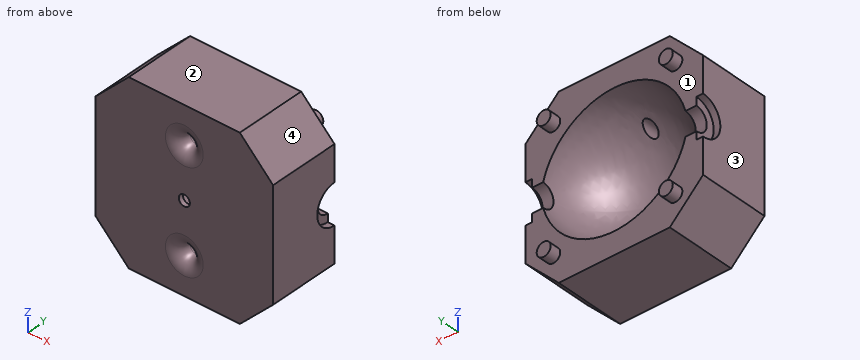
from build123d import *

# Parameters (mm, degrees)
SKETCH1_W           = 80
SKETCH1_H           = 80
BOSS_EXTRUDE1_DEPTH = 32
SKETCH3_R           = 5.375
CUT_EXTRUDE1_DEPTH  = 95.994736856
CHAMFER1_SIZE       = 15
SKETCH5_R           = 9
CUT_EXTRUDE3_DEPTH  = 93.482430925
SKETCH4_R           = 3.15
BOSS_EXTRUDE3_DEPTH = 5
CUT_EXTRUDE4_REACH  = 69.594
SKETCH6_R           = 2.5
FILLET1_R           = 6


with BuildPart() as part:
    # Sketch1 → Boss-Extrude1 (new body)
    with BuildSketch(Plane(origin=(0, 0, 0), x_dir=(1, 0, 0), z_dir=(0, 1, 0))):
        Rectangle(SKETCH1_W, SKETCH1_H)
    extrude(amount=BOSS_EXTRUDE1_DEPTH)

    # Sketch2 → Cut-Revolve1 (revolve, cut)
    with BuildSketch(Plane(origin=(0, 32, 0), x_dir=(1, 0, 0), z_dir=(0, 1, 0))):
        with BuildLine():
            Line((-33, 0), (33, 0))
            ThreePointArc((33, 0), (0, -30), (-33, 0))
        make_face()
    revolve(axis=Axis((-33, 32, 0), (1, 0, 0)), mode=Mode.SUBTRACT)

    # Sketch3 → Cut-Extrude1 (cut, through all)
    with BuildSketch(Plane.ZY.offset(40)):
        with Locations((0, 32)):
            Circle(SKETCH3_R)
    extrude(amount=-CUT_EXTRUDE1_DEPTH, mode=Mode.SUBTRACT)

    # Chamfer1
    chamfer1_edges = [part.edges().sort_by_distance(p)[0] for p in [
        (40, 16, 40),
        (-40, 16, 40),
        (-40, 16, -40),
        (40, 16, -40),
    ]]
    chamfer(chamfer1_edges, length=CHAMFER1_SIZE)

    # Sketch5 → Cut-Extrude3 (cut, through all)
    with BuildSketch(Plane.ZY.offset(37)):
        with Locations((0, 32)):
            Circle(SKETCH5_R)
    cut_extrude3 = extrude(amount=CUT_EXTRUDE3_DEPTH, mode=Mode.SUBTRACT)

    # Mirror1: Cut-Extrude3 across plane
    add(cut_extrude3.mirror(Plane(origin=(0, 0, 0), x_dir=(0, 0, 1), z_dir=(1, 0, 0))), mode=Mode.SUBTRACT)

    # Sketch4 → Boss-Extrude3 (add)
    with BuildSketch(Plane(origin=(0, 32, 0), x_dir=(1, 0, 0), z_dir=(0, 1, 0))):
        with Locations(Location((-27.5, 27.5, 0), (0, 0, 270))):
            Circle(SKETCH4_R)
        with Locations(Location((27.5, 27.5, 0), (0, 0, 270))):
            Circle(SKETCH4_R)
        with Locations(Location((27.5, -27.5, 0), (0, 0, 270))):
            Circle(SKETCH4_R)
        with Locations(Location((-27.5, -27.5, 0), (0, 0, 270))):
            Circle(SKETCH4_R)
    extrude(amount=BOSS_EXTRUDE3_DEPTH)

    # Sketch6 → Cut-Extrude4 (cut, up to next)
    with BuildSketch(Plane.XZ, mode=Mode.PRIVATE) as cut_extrude4_sk1:
        with Locations(Location((0, -23, 0), (0, 0, 270))):
            Circle(SKETCH6_R)
    cut_extrude4_tool1 = extrude(cut_extrude4_sk1.sketch, amount=-CUT_EXTRUDE4_REACH, mode=Mode.PRIVATE) & part.part
    # Sketch6 → Cut-Extrude4 (cut, up to next)
    with BuildSketch(Plane.XZ, mode=Mode.PRIVATE) as cut_extrude4_sk2:
        with Locations(Location((0, 23, 0), (0, 0, 229.659534443))):
            Circle(SKETCH6_R)
    cut_extrude4_tool2 = extrude(cut_extrude4_sk2.sketch, amount=-CUT_EXTRUDE4_REACH, mode=Mode.PRIVATE) & part.part
    # Sketch6 → Cut-Extrude4 (cut, up to next)
    with BuildSketch(Plane.XZ, mode=Mode.PRIVATE) as cut_extrude4_sk3:
        with Locations(Location((0, 0, 0), (0, 0, 270))):
            Circle(SKETCH6_R)
    cut_extrude4_tool3 = extrude(cut_extrude4_sk3.sketch, amount=-CUT_EXTRUDE4_REACH, mode=Mode.PRIVATE) & part.part
    add(cut_extrude4_tool1.solids().sort_by_distance((0, 0, -23))[0], mode=Mode.SUBTRACT)
    add(cut_extrude4_tool2.solids().sort_by_distance((0, 0, 23))[0], mode=Mode.SUBTRACT)
    add(cut_extrude4_tool3.solids().sort_by_distance((0, 0, 0))[0], mode=Mode.SUBTRACT)

    # Fillet1
    fillet1_edges = [part.edges().sort_by_distance(p)[0] for p in [
        (0, 0, -20.5),
        (1.618320645, 0, 24.905528349),
    ]]
    fillet(fillet1_edges, radius=FILLET1_R)


solid = part.part
Read the model definition and answer for the solid it produces. Units are mm, in the model's axes. Face numbers are marked on the shaded views. Give positions to 0.01 mm unless a question says otherwise; leave off trailing zeros. Write each loop counter-clockwise with the first axis right and the second up, starting at its lowest first coordinate (ties: lowest second). Pieces come first, ordered by that corner, then holes. Notation, with made-up numbers: M 1.25,26.25 L 17.25,26.25 A32 cw 17.25,55.25 Z; hole C 11,-26.5 d6. An arc over 180 degrees is marked long. One line per item, written item: value. Start each with the question number.
(1) Find section A-A (x = 33). Determine the outline of the cut face in (y, z) (3 decimals), plus the area to 3 significant figures.
(2) Find the intervals of material crossed by line 1 (X direction, y = 9, z = -23); line 2 (Z direction, x = 0, y = 11); line 3 (Z direction, x = 6.5, y = 25.5), in increasing order.
(3) Determine the mould class of the marked faces 1, 2, 3 and 4 for opening direction X: pulls with the +X half, pulls with the -X half, needs draft (parallel to the pull), parting line crosses it, or undercut.
(4) Flat-ended cylindrical pins translate along their axes: pin 1 Ø10 at (y, z) = (27, -4.5) entering from -X; pin 2 Ø2 at (x, z) = (8, -18.5) entering from +Y; pin 3 Ø6.5 at (x, z) = (0, 0) entering from +Y; pin 4 Ø4.5 at (y, z) = (29, -1) entering from +X. Find the tip coordinate at first contact, or state that the pin passes through.
(5) Find section B-B (y = 8). Give the number of separate pieces and of enclosed holes in the cut face, plus the area to 3 significant figures.
Results below:
1. outline: M 0,-32 L 32,-32 L 32,-5.375 A5.375 cw 32,5.375 L 32,32 L 0,32 Z
1. area: 2,000 mm^2
2. line 1: x = -40 to -2.5, 2.5 to 40
2. line 2: z = -40 to -25.5, 25.5 to 40
2. line 3: z = -40 to -28.63, 28.63 to 40
3. face 1: undercut
3. face 2: needs draft
3. face 3: pulls with the -X half
3. face 4: pulls with the +X half
4. pin 1: stops at x = -40
4. pin 2: stops at y = 10.57
4. pin 3: stops at y = 2.18
4. pin 4: stops at x = 37
5. separate pieces: 1
5. enclosed holes: 3
5. area: 4,840 mm^2
